For this review, take the finished solid that the model builds, in its own axes (mm). Face numbers are marked on the shaded views. A direction names the side the tool comes from. Give positions to 0.01 mm unless a question says otherwise; leave off trailing zeros. Order: outer loops, then holes, each group sorted by start corner. A loop starts at its lowest first (then second) coordinate and runs counter-clockwise, first axis right, second up. Notation, with made-up numbers: (31.5, 37) -> (90.5, 37) arc R8 ccw to (90.5, 50) -> close; hole circle Ø10 at (38, 49). An arc over 180 degrees is marked (long way). Use CSV: the item, a comma, the result in double quotes. Start each with the question number.
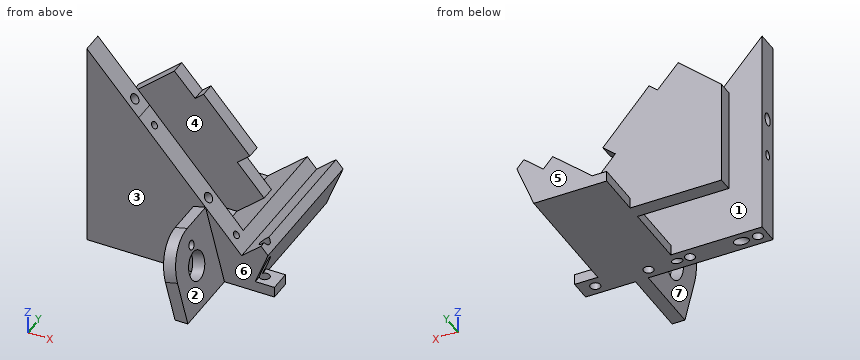
```python
from build123d import *

# Parameters (mm, degrees)
ESQUISSE4_W             = 52.781616476
ESQUISSE4_H             = 6
BOSS_EXTRU_1_DEPTH      = 3
BOSS_EXTRU_2_DEPTH      = 41
ENL_V_MAT_EXTRU_1_DEPTH = 35
BOSS_EXTRU_3_DEPTH      = 4
ESQUISSE11_R            = 1.4
ENL_V_MAT_EXTRU_2_DEPTH = 43
BOSS_EXTRU_4_DEPTH      = 41
ESQUISSE15_R            = 1
ENL_V_MAT_EXTRU_4_DEPTH = 30
BOSS_EXTRU_5_DEPTH      = 20
ESQUISSE18_R            = 4
ENL_V_MAT_EXTRU_5_DEPTH = 12
ESQUISSE12_R            = 1.4
ENL_V_MAT_EXTRU_6_DEPTH = 18
ESQUISSE19_R            = 1.254640732
ENL_V_MAT_EXTRU_7_DEPTH = 18
CONG_1_R                = 10
ESQUISSE20_W            = 12.811790935
ESQUISSE20_H            = 3
BOSS_EXTRU_7_DEPTH      = 36


with BuildPart() as part:
    # Esquisse4 → Boss.-Extru.1 (new body)
    with BuildSketch(Plane.XY):
        with Locations((48.08341362, -51.85)):
            Rectangle(ESQUISSE4_W, ESQUISSE4_H)
    extrude(amount=BOSS_EXTRU_1_DEPTH)

    # Esquisse6 → Boss.-Extru.2 (add)
    with BuildSketch(Plane.XZ.offset(54.85)):
        Polygon((65.242227071, 9.760964304), (70.700086364, 14.539666718), (72.676320449, 12.282567065), (62.07450001, 3), (21.692605382, 3), (21.692605382, 29.804497378), (21.692605382, 59.423332345), (36.271065294, 42.849554228), align=None)
    extrude(amount=-BOSS_EXTRU_2_DEPTH)

    # Esquisse9 → Enlèv. mat.-Extru.1 (cut)
    with BuildSketch(Plane(origin=(0, -13.85, 0), x_dir=(1, 0, 0), z_dir=(0, 1, 0))):
        Polygon((36.271065294, -42.849554228), (62.613078874, -12.763771276), (51.461664708, -3), (21.692605382, -3), (21.692605382, -29.804497378), (21.692605382, -59.423332345), align=None)
    extrude(amount=-ENL_V_MAT_EXTRU_1_DEPTH, mode=Mode.SUBTRACT)

    # Esquisse10 → Boss.-Extru.3 (add)
    with BuildSketch(Plane(origin=(0, -26.644686639, 0), x_dir=(1, 0, 0), z_dir=(0, 1, 0))):
        Polygon((42.072152074, -36.224007657), (39.690998774, -34.139156727), (33.841851451, -40.675851871), (21.692605382, -29.804497378), (21.692605382, 0), (48.035299878, 0), (59.09491831, -9.68339828), (51.563800233, -18.28485098), (55.081960797, -21.365223976), align=None)
    extrude(amount=-BOSS_EXTRU_3_DEPTH)

    # Esquisse11 → Enlèv. mat.-Extru.2 (cut)
    with BuildSketch(Plane(origin=(41.768421189, 0, 36.570905264), x_dir=(0.658744695, 0, -0.752366551), z_dir=(0.752366551, 0, 0.658744695))):
        with Locations((19.134147904, -51.85)):
            Circle(ESQUISSE11_R)
        with Locations((-12.365852096, -51.85)):
            Circle(ESQUISSE11_R)
    extrude(amount=-ENL_V_MAT_EXTRU_2_DEPTH, mode=Mode.SUBTRACT)

    # Esquisse13 → Boss.-Extru.4 (add)
    with BuildSketch(Plane.XZ.offset(54.85)):
        Polygon((70.700086364, 14.539666718), (60.213373733, 5.357883848), (60.213373733, 0), (67.941059656, 0), (72.676320449, 12.282567065), align=None)
    extrude(amount=-BOSS_EXTRU_4_DEPTH)

    # Esquisse15 → Enlèv. mat.-Extru.4 (cut)
    with BuildSketch(Plane(origin=(41.768421189, 0, 36.570905264), x_dir=(0.658744695, 0, -0.752366551), z_dir=(0.752366551, 0, 0.658744695))):
        with Locations((31.034147904, -51.85)):
            Circle(ESQUISSE15_R)
        with Locations((-3.965852096, -51.85)):
            Circle(ESQUISSE15_R)
    extrude(amount=-ENL_V_MAT_EXTRU_4_DEPTH, mode=Mode.SUBTRACT)

    # Esquisse16 → Boss.-Extru.5 (add)
    with BuildSketch(Plane(origin=(0, -54.85, 0), x_dir=(1, 0, 0), z_dir=(0, 1, 0))):
        Polygon((60.41759692, 0), (55.081960797, -21.365223976), (51.686250118, -20.517197455), (56.810104658, 0), align=None)
    extrude(amount=-BOSS_EXTRU_5_DEPTH)

    # Esquisse18 → Enlèv. mat.-Extru.5 (cut)
    with BuildSketch(Plane(origin=(56.870719104, 0, 14.202587508), x_dir=(0.242293292, 0, -0.970203051), z_dir=(0.970203051, 0, 0.242293292))):
        with Locations((3.628081272, -64.85)):
            Circle(ESQUISSE18_R)
    extrude(amount=-ENL_V_MAT_EXTRU_5_DEPTH, mode=Mode.SUBTRACT)

    # Esquisse12 → Enlèv. mat.-Extru.6 (cut)
    with BuildSketch(Plane(origin=(0, 0, 0), x_dir=(-1, 0, 0), z_dir=(0, 0, -1))):
        with Locations((-24.42996151, -51.85)):
            Circle(ESQUISSE12_R)
        with Locations((-43.52996151, -51.85)):
            Circle(ESQUISSE12_R)
        with Locations((-55.197893581, -51.85)):
            Circle(ESQUISSE12_R)
        with Locations((-70.197893581, -51.85)):
            Circle(ESQUISSE12_R)
    extrude(amount=-ENL_V_MAT_EXTRU_6_DEPTH, mode=Mode.SUBTRACT)

    # Esquisse19 → Enlèv. mat.-Extru.7 (cut)
    with BuildSketch(Plane(origin=(56.870719104, 0, 14.202587508), x_dir=(0.242293292, 0, -0.970203051), z_dir=(0.970203051, 0, 0.242293292))):
        with Locations((-2.43609109, -64.85)):
            Circle(ESQUISSE19_R)
    extrude(amount=-ENL_V_MAT_EXTRU_7_DEPTH, mode=Mode.SUBTRACT)

    # Congé1
    cong_1_edges = [part.edges().sort_by_distance(p)[0] for p in [
        (53.384105458, -74.85, 20.941210715),
    ]]
    fillet(cong_1_edges, radius=CONG_1_R)

    # Esquisse20 → Boss.-Extru.7 (add)
    with BuildSketch(Plane(origin=(0, -13.85, 0), x_dir=(1, 0, 0), z_dir=(0, 1, 0))):
        with Locations((53.807478266, -1.5)):
            Rectangle(ESQUISSE20_W, ESQUISSE20_H)
    extrude(amount=-BOSS_EXTRU_7_DEPTH)


solid = part.part
```
1. Consider section A-A (y = -32). State the section outline as (x, z) points, plus the area to 3 significant figures.
2. For the marked faces 5, 6 and 7, list the 3-axis set-ups (+Z, -Z, +X, -X, +Y, -Y) from which the entire face can be reached by the end or side of a thin tool; tool diameter is ignored.
3. Consider section B-B (y = -62). State the section outline as (x, z) points, plus the area to 3 significant figures.
4. Draft analysis for pull direction Y (two halves, no side actions). For the marked faces 1, 2, 3 and 4, state which applies: +Y half, -Y half, draft (parallel to the pull), parting line (faces both ways), or undercut.
5. Consider section C-C (y = -51.85). State how many separate pieces and enclosed holes the cut face has, plus the area to 3 significant figures.
6. Clearance check with flat-ended pins moving along their axes: P1, Ø0.8, axis at x = 55, y = -51.5, coming from the -Z side; P2, Ø1.7, axis at x = 24.43, y = -51.85, coming from the +Z side; P3, Ø4, axis at y = -45.5, z = 14.5, coming from the +X side; P4, Ø2.5, axis at x = 70.2, y = -51.85, coming from the -Z side. State where each tip first meets the part, or that it passes through.
7. To check wall thickness, follow L1, parallel to Y at x = 30, z = 22.5; L2, parallel to Y at x = 51, z = 18; L3, parallel to Z at x = 48, y = -17. State the ranges of each line that lie inside material, in increasing order. Write a range as [from, to].
Answer list:
1,outline,"(47.4, 0) -> (67.94, 0) -> (72.68, 12.28) -> (70.7, 14.54) -> (65.24, 9.76) -> (62.61, 12.76) -> (51.46, 3) -> (47.4, 3) -> close"
1,area,"193 mm2"
2,face 5,"+Z, -Z, +X, -X, +Y"
2,face 6,"+Z, +X, -Y"
2,face 7,"-Z, -X, -Y"
3,outline,"(51.69, 20.52) -> (53.67, 12.56) -> (57.07, 13.41) -> (55.08, 21.37) -> close; (55.03, 7.11) -> (56.81, 0) -> (60.42, 0) -> (58.43, 7.96) -> close"
3,area,"55.9 mm2"
4,face 1,"undercut"
4,face 2,"draft"
4,face 3,"-Y half"
4,face 4,"undercut"
5,separate pieces,"9"
5,enclosed holes,"0"
5,area,"1,200 mm2"
6,P1,"z = 18"
6,P2,"z = 57.28"
6,P3,"x = 72.49"
6,P4,"through"
7,L1,"[-54.85, -48.85], [-30.64, -26.64]"
7,L2,"[-54.85, -52.91], [-50.79, -48.85], [-30.64, -26.64]"
7,L3,"[0, 3]"
